Read the model definition and answer for the solid it produces. Units are mm, in the model's axes. Face numbers are marked on the shaded views. A direction names the side the tool comes from. Give positions to 0.01 mm unless a question says otherwise; leave off trailing zeros. Loops run counter-clockwise (first coordinate to the right, second up) from the corner with the lowest first, then second, coordinate; pieces in that order, holes last. Notation, with made-up numbers: (-24.75, 17.5) -> (19.25, 17.5) arc R16 ccw to (19.25, 43.5) -> close; hole circle Ø7 at (28, -28.75). An arc over 180 degrees is marked (long way). Write each question's results on one line, items separated by ' | '. Start each with the question number.
Item 1: Determine the mould class of the marked faces 1, 2, 3 and 4 for opening direction Z: +Z half, -Z half, draft (parallel to the pull), parting line (faces both ways), or undercut.
Item 2: Section D-D on z = -104 is taken. Write down the section's boundary in (x, y).
Item 3: Which of the six approach directions +Z, -Z, +X, -X, +Y, -Y give full straight-line access (tool end or side, diameter ignored) to the marked faces 5 and 6?
Item 4: Section C-C on y = 137 is taken. Write down the section's boundary in (x, z).
Item 5: Section B-B on y = 17 is taken. Write down the section's boundary in (x, z).
Item 6: Find the intervals of material crossed by line 1 (Z direction, x = -209.5, y = 126.5); line 2 (Z direction, x = -255, y = 86.5); line 3 (X direction, y = 70, z = -26), in increasing order.
Item 7: Each of these flat-tipped pins is pushed along its axis until it touches: P1, Ø8, axis at x = -269, y = 121, coming from the -Z side; P2, Ø10.5, axis at x = -130.5, y = 28.34, coming from the +Z side; P3, Ø10, axis at y = 114.5, z = -98.5, coming from the -X side. Where does it stop, or does it pass through?
Item 8: Section A-A on x = -143.5 is taken. Write down the section's boundary in (y, z).
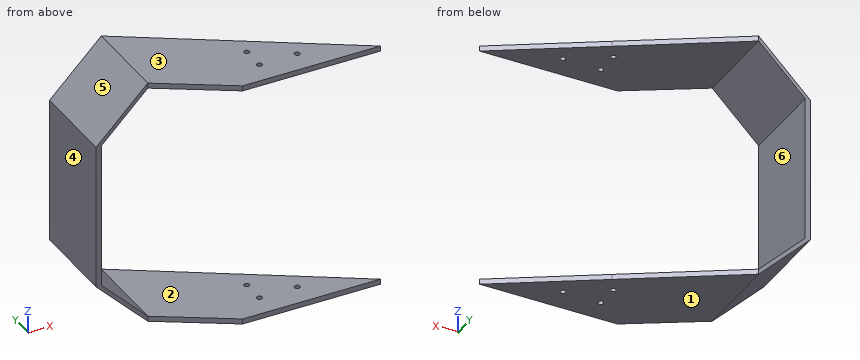
```python
from build123d import *

# Parameters (mm, degrees)
SKETCH5_W                = 6.35
SKETCH5_H                = 176
BOSS_EXTRUDE1_DEPTH      = 104.775666
BOSS_EXTRUDE2_DEPTH      = 6.35
BOSS_EXTRUDE3_DEPTH      = 6.35
M6_CLEARANCE_HOLE5_D     = 6.6
M6_CLEARANCE_HOLE5_DEPTH = 6.35
M6_CLEARANCE_HOLE4_D     = 6.6


with BuildPart() as part:
    # Sketch5 → Boss-Extrude1 (new body)
    with BuildSketch(Plane(origin=(0, 52.149159956, 0), x_dir=(1, 0, 0), z_dir=(0, 1, 0))):
        with Locations((-311.081896744, 0)):
            Rectangle(SKETCH5_W, SKETCH5_H)
        Polygon((-252.0315, -143.875396744), (-307.906896744, -88), (-314.256896744, -88), (-252.0315, -150.225396744), align=None)
        Polygon((-307.906896744, 88), (-252.0315, 143.875396744), (-252.0315, 150.225396744), (-314.256896744, 88), align=None)
    extrude(amount=BOSS_EXTRUDE1_DEPTH)

    # Sketch3 → Boss-Extrude2 (add)
    with BuildSketch(Plane.XY.offset(150.225396744)):
        Polygon((-130.499303898, 0), (-39.48466449, 0), (-84.991984194, 28.335711553), (-130.499303898, 28.335711553), align=None)
        Polygon((-39.48466449, 0), (0, 0), (-119.473415555, 74.388895455), (-165.790897492, 0), (-130.499303898, 0), (-130.499303898, 28.335711553), (-130.499303898, 56.671423106), (-84.991984194, 28.335711553), align=None)
        Polygon((-165.790897492, 0), (-119.473415555, 74.388895455), (-165.790897492, 103.228), align=None)
        Polygon((-130.499303898, 28.335711553), (-84.991984194, 28.335711553), (-130.499303898, 56.671423106), align=None)
        Polygon((-165.790897492, 0), (-165.790897492, 103.228), (-252.0315, 156.924825642), (-252.0315, 52.149159956), align=None)
    extrude(amount=-BOSS_EXTRUDE2_DEPTH)

    # Sketch8 → Boss-Extrude3 (add)
    with BuildSketch(Plane.XY.offset(-150.225396744)):
        Polygon((-165.790897492, 0), (-165.790897492, 103.228), (-252.0315, 156.924825642), (-252.0315, 52.149159956), align=None)
        Polygon((-165.790897492, 0), (-119.473415555, 74.388895455), (-165.790897492, 103.228), align=None)
        Polygon((-39.48466449, 0), (0, 0), (-119.473415555, 74.388895455), (-165.790897492, 0), (-130.499303898, 0), (-130.499303898, 28.335711553), (-130.499303898, 56.671423106), (-84.991984194, 28.335711553), align=None)
        Polygon((-130.499303898, 0), (-39.48466449, 0), (-84.991984194, 28.335711553), (-130.499303898, 28.335711553), align=None)
        Polygon((-130.499303898, 28.335711553), (-84.991984194, 28.335711553), (-130.499303898, 56.671423106), align=None)
    extrude(amount=BOSS_EXTRUDE3_DEPTH)

    # M6 Clearance Hole5
    with Locations(Plane(origin=(0, 0, -150.225396744), x_dir=(1, 0, 0), z_dir=(0, 0, -1))):
        with Locations((-84.991984194, -28.335711553), (-130.499303898, -28.335711553), (-130.499303898, -56.671423106)):
            Hole(M6_CLEARANCE_HOLE5_D / 2, depth=M6_CLEARANCE_HOLE5_DEPTH)

    # M6 Clearance Hole4 (through all)
    with Locations(Plane.XY.offset(150.225396744)):
        with Locations((-84.991984194, 28.335711553), (-130.499303898, 28.335711553), (-130.499303898, 56.671423106)):
            Hole(M6_CLEARANCE_HOLE4_D / 2)


solid = part.part
```
Findings:
1) face 1: -Z half | face 2: undercut | face 3: +Z half | face 4: draft
2) outline: (-298.26, 52.15) -> (-291.91, 52.15) -> (-291.91, 156.92) -> (-298.26, 156.92) -> close
3) face 5: +Z, -X, +Y, -Y | face 6: +X, +Y, -Y
4) outline: (-314.26, -88) -> (-252.03, -150.23) -> (-220.03, -150.23) -> (-220.03, -143.88) -> (-252.03, -143.88) -> (-307.91, -88) -> (-307.91, 88) -> (-252.03, 143.88) -> (-220.03, 143.88) -> (-220.03, 150.23) -> (-252.03, 150.23) -> (-314.26, 88) -> close
5) outline: (-193.9, -150.23) -> (-27.3, -150.23) -> (-27.3, -143.88) -> (-193.9, -143.88) -> close; (-193.9, 143.88) -> (-27.3, 143.88) -> (-27.3, 150.23) -> (-193.9, 150.23) -> close
6) line 1: -150.23 to -143.88, 143.88 to 150.23 | line 2: -147.26 to -140.91, 140.91 to 147.26 | line 3: -314.26 to -307.91
7) P1: z = -137.26 | P2: z = 150.23 | P3: x = -308.76
8) outline: (0, -150.23) -> (89.35, -150.23) -> (89.35, -143.88) -> (0, -143.88) -> close; (0, 143.88) -> (89.35, 143.88) -> (89.35, 150.23) -> (0, 150.23) -> close
